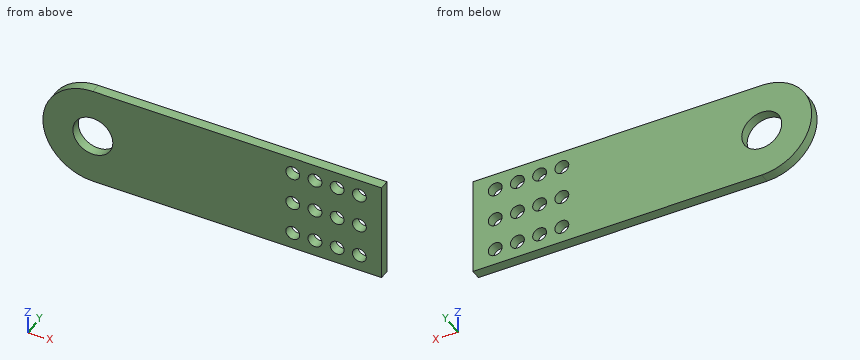
from build123d import *

# Parameters (mm, degrees)
SKETCH1_R                     = 9
BOSS_EXTRUDE1_DEPTH           = 2.25
CUT_EXTRUDE1_START            = -5.5
SKETCH2_R                     = 3.125
CUT_EXTRUDE1_DEPTH            = 6.5
LPATTERN1_COUNT               = 4
LPATTERN1_PITCH               = 10
LPATTERN2_COUNT               = 2
LPATTERN2_PITCH               = 15
LPATTERN2_START               = -5.5
LPATTERN2_COPY_1_SKETCH_R     = 3.125
LPATTERN2_COPY_1_DEPTH        = 6.5
LPATTERN2_COPY_2_SKETCH_R     = 3.125
LPATTERN2_COPY_2_DEPTH        = 6.5
LPATTERN2_COPY_3_SKETCH_R     = 3.125
LPATTERN2_COPY_3_DEPTH        = 6.5
LPATTERN2_COL_COUNT           = 2
LPATTERN2_COL_PITCH           = 15
LPATTERN2_COL_COPY_1_SKETCH_R = 3.125
LPATTERN2_COL_COPY_1_DEPTH    = 6.5
LPATTERN2_COL_COPY_2_SKETCH_R = 3.125
LPATTERN2_COL_COPY_2_DEPTH    = 6.5
LPATTERN2_COL_COPY_3_SKETCH_R = 3.125
LPATTERN2_COL_COPY_3_DEPTH    = 6.5
CUT_EXTRUDE2_DEPTH            = 1
CUT_EXTRUDE2_DEPTH_BACK       = 5.5


with BuildPart() as part:
    # Sketch1 → Boss-Extrude1 (new body, symmetric)
    with BuildSketch(Plane(origin=(0, 0, 0), x_dir=(1, 0, 0), z_dir=(0, 1, 0))):
        Polygon((130, -22.5), (0, -22.5), (-30, -22.5), (-30, 22.5), (0, 22.5), (130, 22.5), align=None)
        Circle(SKETCH1_R, mode=Mode.SUBTRACT)
    extrude(amount=BOSS_EXTRUDE1_DEPTH, both=True)

    # Sketch2 → Cut-Extrude1 (cut)
    with BuildSketch(Plane(origin=(0, 2.25, 0), x_dir=(1, 0, 0), z_dir=(0, 1, 0)).offset(CUT_EXTRUDE1_START)):
        with Locations((120, 0)):
            Circle(SKETCH2_R)
    cut_extrude1 = extrude(amount=CUT_EXTRUDE1_DEPTH, mode=Mode.SUBTRACT)

    # LPattern1: Cut-Extrude1 ×4
    with Locations(*[(-i * LPATTERN1_PITCH, 0, 0) for i in range(1, LPATTERN1_COUNT)]):
        add(cut_extrude1, mode=Mode.SUBTRACT)

    # LPattern2: Cut-Extrude1 ×2
    with Locations(*[(0, 0, i * LPATTERN2_PITCH) for i in range(1, LPATTERN2_COUNT)]):
        add(cut_extrude1, mode=Mode.SUBTRACT)

    # LPattern2 copy 1 sketch → LPattern2 copy 1 (cut)
    with BuildSketch(Plane(origin=(-10, 2.25, 15), x_dir=(1, 0, 0), z_dir=(0, 1, 0)).offset(LPATTERN2_START)):
        with Locations((120, 0)):
            Circle(LPATTERN2_COPY_1_SKETCH_R)
    extrude(amount=LPATTERN2_COPY_1_DEPTH, mode=Mode.SUBTRACT)

    # LPattern2 copy 2 sketch → LPattern2 copy 2 (cut)
    with BuildSketch(Plane(origin=(-20, 2.25, 15), x_dir=(1, 0, 0), z_dir=(0, 1, 0)).offset(LPATTERN2_START)):
        with Locations((120, 0)):
            Circle(LPATTERN2_COPY_2_SKETCH_R)
    extrude(amount=LPATTERN2_COPY_2_DEPTH, mode=Mode.SUBTRACT)

    # LPattern2 copy 3 sketch → LPattern2 copy 3 (cut)
    with BuildSketch(Plane(origin=(-30, 2.25, 15), x_dir=(1, 0, 0), z_dir=(0, 1, 0)).offset(LPATTERN2_START)):
        with Locations((120, 0)):
            Circle(LPATTERN2_COPY_3_SKETCH_R)
    extrude(amount=LPATTERN2_COPY_3_DEPTH, mode=Mode.SUBTRACT)

    # LPattern2 col: Cut-Extrude1 ×2
    with Locations(*[(0, 0, -i * LPATTERN2_COL_PITCH) for i in range(1, LPATTERN2_COL_COUNT)]):
        add(cut_extrude1, mode=Mode.SUBTRACT)

    # LPattern2 col copy 1 sketch → LPattern2 col copy 1 (cut)
    with BuildSketch(Plane(origin=(-10, 2.25, -15), x_dir=(1, 0, 0), z_dir=(0, 1, 0)).offset(LPATTERN2_START)):
        with Locations((120, 0)):
            Circle(LPATTERN2_COL_COPY_1_SKETCH_R)
    extrude(amount=LPATTERN2_COL_COPY_1_DEPTH, mode=Mode.SUBTRACT)

    # LPattern2 col copy 2 sketch → LPattern2 col copy 2 (cut)
    with BuildSketch(Plane(origin=(-20, 2.25, -15), x_dir=(1, 0, 0), z_dir=(0, 1, 0)).offset(LPATTERN2_START)):
        with Locations((120, 0)):
            Circle(LPATTERN2_COL_COPY_2_SKETCH_R)
    extrude(amount=LPATTERN2_COL_COPY_2_DEPTH, mode=Mode.SUBTRACT)

    # LPattern2 col copy 3 sketch → LPattern2 col copy 3 (cut)
    with BuildSketch(Plane(origin=(-30, 2.25, -15), x_dir=(1, 0, 0), z_dir=(0, 1, 0)).offset(LPATTERN2_START)):
        with Locations((120, 0)):
            Circle(LPATTERN2_COL_COPY_3_SKETCH_R)
    extrude(amount=LPATTERN2_COL_COPY_3_DEPTH, mode=Mode.SUBTRACT)

    # Sketch3 → Cut-Extrude2 (cut, two sides)
    with BuildSketch(Plane(origin=(0, 2.25, 0), x_dir=(1, 0, 0), z_dir=(0, 1, 0))) as cut_extrude2_sk:
        with BuildLine():
            ThreePointArc((-4.9e-08, -22.5), (-22.5, 2.1e-08), (-7e-09, 22.5))
            Line((-7e-09, 22.5), (-30, 22.5))
            Line((-30, 22.5), (-30, -22.5))
            Line((-30, -22.5), (-4.9e-08, -22.5))
        make_face()
    extrude(amount=CUT_EXTRUDE2_DEPTH, mode=Mode.SUBTRACT)
    extrude(cut_extrude2_sk.sketch, amount=-CUT_EXTRUDE2_DEPTH_BACK, mode=Mode.SUBTRACT)


solid = part.part
The model under review builds one solid part; all positions refer to its coordinate system, in mm. Round coordinates to 2 decimals unless told otherwise and drop trailing zeros. Loops run counter-clockwise (first coordinate to the right, second up) from the corner with the lowest first, then second, coordinate; pieces in that order, holes last. Notation, with made-up numbers: (-25, -6.75) -> (28, -6.75) arc R18 cw to (28, 24.25) -> close; hole circle Ø6 at (87.5, 35.5). An arc over 180 degrees is marked (long way). Write item = value, one per line. Start each with the question number.
Item 1: Take a section at B-B on y = 1.05. Count the separate pieces of the cut face and the enclosed holes in it, plus the area to 3 significant figures.
Item 2: Take a section at C-C on z = -5. Give the boundary of the cut face in (x, y).
Item 3: Take a section at A-A on x = 90. Give the boundary of the cut face in (y, z) (3 decimals).
Item 4: To check wall thickness, follow L1, parallel to Z at x = 110, y = -1.2 (3 decimals); L2, parallel to X at y = 0.3, z = -1; L3, parallel to X at y = -0.4, z = 16.5. State the ranges of each line that lie inside material, in increasing order.
Item 5: Take a section at D-D on x = 2.5. Give the boundary of the cut face in (y, z).
Item 6: Insertion check: pin 1 (5.5 mm diameter, centred on x = 90, z = 15, fed in from +Y); pin 2 (1.5 mm diameter, centred on y = 0, z = -12, fed in from -X). Each pin has a flat end and moves straight along its axis. Give the tip position at first contact, or say it passes through.
Result:
q1.separate_pieces = 1
q1.enclosed_holes = 13
q1.area = 6,020 mm²
q2.outline = (-21.94, -2.25) -> (-7.48, -2.25) -> (-7.48, 2.25) -> (-21.94, 2.25) -> close; (7.48, -2.25) -> (130, -2.25) -> (130, 2.25) -> (7.48, 2.25) -> close
q3.outline = (-2.25, -22.5) -> (2.25, -22.5) -> (2.25, -18.125) -> (-2.25, -18.125) -> close; (-2.25, -11.875) -> (2.25, -11.875) -> (2.25, -3.125) -> (-2.25, -3.125) -> close; (-2.25, 3.125) -> (2.25, 3.125) -> (2.25, 11.875) -> (-2.25, 11.875) -> close; (-2.25, 18.125) -> (2.25, 18.125) -> (2.25, 22.5) -> (-2.25, 22.5) -> close
q4.L1 = -22.5 to -18.125, -11.875 to -3.125, 3.125 to 11.875, 18.125 to 22.5
q4.L2 = -22.48 to -8.94, 8.94 to 87.04, 92.96 to 97.04, 102.96 to 107.04, 112.96 to 117.04, 122.96 to 130
q4.L3 = -15.3 to 87.26, 92.74 to 97.26, 102.74 to 107.26, 112.74 to 117.26, 122.74 to 130
q5.outline = (-2.25, -22.5) -> (2.25, -22.5) -> (2.25, -8.65) -> (-2.25, -8.65) -> close; (-2.25, 8.65) -> (2.25, 8.65) -> (2.25, 22.5) -> (-2.25, 22.5) -> close
q6.pin_1 = through
q6.pin_2 = -19.49
